```python
from build123d import *

# Parameters (mm, degrees)
BOSS_EXTRUDE2_DEPTH = 6.35
SKETCH2_R           = 3.175
CUT_EXTRUDE1_DEPTH  = 7.35
SKETCH5_R           = 4.6625
BOSS_EXTRUDE3_DEPTH = 12.7
SKETCH6_W           = 177.8
SKETCH6_H           = 6.35
CUT_EXTRUDE2_DEPTH  = 3.175
SKETCH7_R           = 2.286
CUT_EXTRUDE3_DEPTH  = 12.7
SKETCH8_R           = 2.286
CUT_EXTRUDE4_DEPTH  = 20.05
SKETCH9_R           = 2.286
CUT_EXTRUDE5_DEPTH  = 20.05


with BuildPart() as part:
    # Sketch1 → Boss-Extrude2 (new body)
    with BuildSketch(Plane(origin=(0, 0, 0), x_dir=(1, 0, 0), z_dir=(0, 1, 0))):
        with BuildLine():
            Line((0, 0), (0, 25.4))
            ThreePointArc((0, 25.4), (3.719743879, 34.380256121), (12.7, 38.1))
            Line((12.7, 38.1), (190.5, 38.1))
            ThreePointArc((190.5, 38.1), (199.480256121, 34.380256121), (203.2, 25.4))
            Line((203.2, 25.4), (203.2, -152.4))
            ThreePointArc((203.2, -152.4), (199.480256121, -161.380256121), (190.5, -165.1))
            Line((190.5, -165.1), (12.7, -165.1))
            ThreePointArc((12.7, -165.1), (3.719743879, -161.380256121), (0, -152.4))
            Line((0, -152.4), (0, -127))
            Line((0, -127), (177.8, -127))
            Line((177.8, -127), (177.8, 0))
            Line((177.8, 0), (0, 0))
        make_face()
    extrude(amount=BOSS_EXTRUDE2_DEPTH)

    # Sketch2 → Cut-Extrude1 (cut, through all)
    with BuildSketch(Plane(origin=(0, 6.35, 0), x_dir=(1, 0, 0), z_dir=(0, 1, 0))):
        with Locations((12.7, 25.4)):
            Circle(SKETCH2_R)
        with Locations((190.5, 25.4)):
            Circle(SKETCH2_R)
        with Locations((190.5, -152.4)):
            Circle(SKETCH2_R)
        with Locations((12.7, -152.4)):
            Circle(SKETCH2_R)
    extrude(amount=-CUT_EXTRUDE1_DEPTH, mode=Mode.SUBTRACT)

    # Sketch5 → Boss-Extrude3 (add)
    with BuildSketch(Plane.XZ):
        with Locations((28.575, 136.525)):
            Circle(SKETCH5_R)
        with Locations((174.625, 136.525)):
            Circle(SKETCH5_R)
        with Locations((174.625, -9.525)):
            Circle(SKETCH5_R)
        with Locations((28.575, -9.525)):
            Circle(SKETCH5_R)
    extrude(amount=BOSS_EXTRUDE3_DEPTH)

    # Sketch6 → Cut-Extrude2 (cut)
    with BuildSketch(Plane(origin=(0, 6.35, 0), x_dir=(1, 0, 0), z_dir=(0, 1, 0))):
        with Locations((88.9, -130.175)):
            Rectangle(SKETCH6_W, SKETCH6_H)
        with Locations((88.9, 3.175)):
            Rectangle(SKETCH6_W, SKETCH6_H)
    extrude(amount=-CUT_EXTRUDE2_DEPTH, mode=Mode.SUBTRACT)

    # Sketch7 → Cut-Extrude3 (cut)
    with BuildSketch(Plane(origin=(0, 6.35, 0), x_dir=(1, 0, 0), z_dir=(0, 1, 0))):
        with Locations((188.214, -101.092)):
            Circle(SKETCH7_R)
        with Locations((188.214, -91.186)):
            Circle(SKETCH7_R)
        with Locations((188.214, -35.814)):
            Circle(SKETCH7_R)
        with Locations((188.214, -25.908)):
            Circle(SKETCH7_R)
    extrude(amount=-CUT_EXTRUDE3_DEPTH, mode=Mode.SUBTRACT)

    # Sketch8 → Cut-Extrude4 (cut, through all)
    with BuildSketch(Plane(origin=(0, 6.35, 0), x_dir=(1, 0, 0), z_dir=(0, 1, 0))):
        with Locations((101.6, 25.527)):
            Circle(SKETCH8_R)
        with Locations((190.627, -63.5)):
            Circle(SKETCH8_R)
        with Locations((101.6, -152.527)):
            Circle(SKETCH8_R)
    extrude(amount=-CUT_EXTRUDE4_DEPTH, mode=Mode.SUBTRACT)

    # Sketch9 → Cut-Extrude5 (cut, through all)
    with BuildSketch(Plane(origin=(0, 6.35, 0), x_dir=(1, 0, 0), z_dir=(0, 1, 0))):
        with Locations((44.321, 24)):
            Circle(SKETCH9_R)
        with Locations((44.321, -151)):
            Circle(SKETCH9_R)
        with Locations((158.879, -151)):
            Circle(SKETCH9_R)
        with Locations((158.879, 24)):
            Circle(SKETCH9_R)
    extrude(amount=-CUT_EXTRUDE5_DEPTH, mode=Mode.SUBTRACT)


solid = part.part
```
The model under review builds one solid part; all positions refer to its coordinate system, in mm. A direction names the side the tool comes from. Coordinates: 2 decimals unless noted, no trailing zeros. Write each loop counter-clockwise with the first axis right and the second up, starting at its lowest first coordinate (ties: lowest second). Pieces come first, ordered by that corner, then holes.
1) To check wall thickness, follow probe 1 along Z at (x, y) = (12.7, 3.5) (3 decimals); probe 2 along Z at (x, y) = (91, 3.75); probe 3 along X at (y, z) = (1.5, 63.5). State the ranges of each line that lie inside material, in increasing order.
2) The part is to be moulded in two halves that separate along Z. For faces 3 (the face through (88, 3.175, -3)), 4 (the face through (199.38, 3.13, -34.48)), 5 (the face through (159.93, 3.22, 153.03)), 6 (the face through (203.2, 3, 62)), say which applies: pulls with the +Z half, pulls with the -Z half, needs draft (parallel to the pull), parting line crosses it, or undercut.
3) We need section B-B on z = 72.5. State the section outline as (x, y) points, then the cut area to 3 significant figures.
4) We need section C-C on y = -6.75. State the section outline as (x, z) points (1 decimal).
5) We need section A-A on x = 75. State the section outline as (y, z) points (3 decimals), then the cut area to 3 significant figures.
6) Machinability: for faces 1 (the face through (12.29, 3.22, -28.55)), 2 (the face through (178.932, -6.261, 134.739)), which of the approach directions +Z, -Z, +X, -X, +Y, -Y give a long, thin tool a straight path to every point of the face, cutting with its end or side? Answer none if there is none.
7) Clearance check with flat-ended pins moving along their axes: pin 1 Ø7.5 at (x, z) = (190.627, 63.5) entering from +Y; pin 2 Ø1.9 at (x, z) = (108, 130) entering from +Y (3 decimals); pin 3 Ø7 at (y, z) = (3.5, 77) entering from -X; pin 4 Ø3.5 at (x, z) = (158.879, -24) entering from +Y. State where each tip first meets the part, or that it passes through.
Answer list:
1. probe 1: z = -38.1 to -28.575, -22.225 to -6.35, 133.35 to 149.225, 155.575 to 165.1
1. probe 2: z = -38.1 to -6.35, 133.35 to 165.1
1. probe 3: x = 177.8 to 188.34, 192.91 to 203.2
2. face 3: undercut
2. face 4: pulls with the -Z half
2. face 5: undercut
2. face 6: needs draft
3. outline: (177.8, 0) - (203.2, 0) - (203.2, 6.35) - (177.8, 6.35) - close
3. area: 161 mm2
4. outline: circle Ø9.3 at (28.6, -9.5); circle Ø9.3 at (28.6, 136.5); circle Ø9.3 at (174.6, -9.5); circle Ø9.3 at (174.6, 136.5)
5. outline: (0, -38.1) - (6.35, -38.1) - (6.35, -6.35) - (3.175, -6.35) - (3.175, 0) - (0, 0) - close; (0, 127) - (3.175, 127) - (3.175, 133.35) - (6.35, 133.35) - (6.35, 165.1) - (0, 165.1) - close
5. area: 444 mm2
6. face 1: +Y, -Y
6. face 2: -Y
7. pin 1: stops at y = 6.35
7. pin 2: stops at y = 3.175
7. pin 3: stops at x = 177.8
7. pin 4: passes through
